Model file for the job. Use its own axes, mm. A direction names the side the tool comes from. Round coordinates to 2 decimals unless told otherwise and drop trailing zeros. Loops run counter-clockwise (first coordinate to the right, second up) from the corner with the lowest first, then second, coordinate; pieces in that order, holes last. Notation, with made-up numbers: M 82,-8.75 L 122,-8.75 A5 cw 122,-2.75 Z; hole C 74.25,-36.75 d11. An arc over 180 degrees is marked long. Use a Markdown table: item, result. Add a question column.
Q1. Tool access for faces 1 (the face through (9.715, 9.699, 6.084)), 2 (the face through (-9.699, 9.715, 6.084)), 3 (the face through (9.699, -9.715, 6.084)), 4 (the face through (-10, 0, 6)): list every direction of +Z, -Z, +X, -X, +Y, -Y with a clear straight run to the whole face (end or side of a thin tool).
Q2. Cut at A-A (y = 7.5). Give the cut face in (x, z), plus the area to 3 significant figures.
Q3. Probe line 1 (Y direction, x = 8, z = 5.5); line 2 (Z direction, x = 10.25, y = 7). List the from-to ranges inside material, lowest first. Write a range as from..to.
Q4. Cut at B-B (z = 8). Give the cut face in (x, y), plus the area to 3 significant figures.
Q5. Pin check, flat tips, straight feed: pin 1 (5 mm diameter, centred on y = 0, z = 5.5, fed in from -X); pin 2 (3 mm diameter, centred on y = 4, z = 7, fed in from +X); pin 3 (1.5 mm diameter, centred on x = -2, z = 8.5, fed in from -Y). Stop position of each tip, or through.
Autodesk Fusion 360 part; units mm, degrees
sketch "Sketch1" plane through (0, 0, 0) normal (0, 0, 1) x (1, 0, 0)
  line L0 (10, -10) -> (-10, -10)
  line L1 (-10, -10) -> (-10, 10)
  line L2 (-10, 10) -> (10, 10)
  line L3 (10, 10) -> (10, -10)
  line L4 (10, -10) -> (-10, 10) construction
  line L5 (-10, -10) -> (10, 10) construction
  line L6 (11.75, -11.75) -> (-11.75, -11.75)
  line L7 (-11.75, -11.75) -> (-11.75, 11.75)
  line L8 (-11.75, 11.75) -> (11.75, 11.75)
  line L9 (11.75, 11.75) -> (11.75, -11.75)
  line L10 (11.75, -11.75) -> (-11.75, 11.75) construction
  line L11 (-11.75, -11.75) -> (11.75, 11.75) construction
  dimension "d1" = 20
  dimension "d2" = 20
  dimension "d3" = 23.5
  dimension "d4" = 23.5
extrude "Extrude1" add sketch "Sketch1" along normal blind 15 contours L0 L1 L2 L3 | L6 L7 L8 L9
extrude "Extrude2" cut sketch "Sketch1" along normal blind 12
fillet "Fillet1" radius 1 4 edges at (11.75, 11.75, 13.5) (-11.75, 11.75, 13.5) (11.75, -11.75, 13.5) (-11.75, -11.75, 13.5)
fillet "Fillet2" radius 1 4 edges at (-10, 10, 6) (10, 10, 6) (10, -10, 6) (-10, -10, 6)
fillet "Fillet3" radius 1.2 8 edges at (-11.4571, 11.4571, 15) (-11.75, 0, 15) (-11.4571, -11.4571, 15) (0, -11.75, 15) (11.4571, -11.4571, 15) (11.75, 0, 15) (11.4571, 11.4571, 15) (0, 11.75, 15)
Checked values:
| question | item | result |
|---|---|---|
| 1 | face 1 | -Z, +X, +Y |
| 1 | face 2 | -Z, -X, +Y |
| 1 | face 3 | -Z, +X, -Y |
| 1 | face 4 | -Z, -X, +Y, -Y |
| 2 | outline | M -11.75,12 L -10,12 L -10,0 L 10,0 L 10,12 L 11.75,12 L 11.75,13.8 A1.2 ccw 10.55,15 L -10.55,15 A1.2 ccw -11.75,13.8 Z |
| 2 | area | 310 mm^2 |
| 3 | line 1 | y = -10..10 |
| 3 | line 2 | z = 12..15 |
| 4 | outline | M -10,-9 A1 ccw -9,-10 L 9,-10 A1 ccw 10,-9 L 10,9 A1 ccw 9,10 L -9,10 A1 ccw -10,9 Z |
| 4 | area | 399 mm^2 |
| 5 | pin 1 | stops at x = -10 |
| 5 | pin 2 | stops at x = 10 |
| 5 | pin 3 | stops at y = -10 |
